Could you check a few things on this model? Use its own coordinates, in mm. Face numbers are marked on the shaded views. Give positions to 0.01 mm unless a question says otherwise; leave off trailing zeros. Write each loop counter-clockwise with the first axis right and the second up, starting at its lowest first coordinate (ties: lowest second). Pieces come first, ordered by that corner, then holes. Notation, with made-up numbers: (15, 65.5) - (49, 65.5) arc R18 ccw to (49, 97.5) - close; hole circle Ø9 at (19, 48). An arc over 180 degrees is marked (long way). Use one line per item in the form item = value.
Autodesk Inventor part; units mm, degrees
ref_plane "Work Plane2" through (0, 202, 0) normal (0, 1, 0) x (1, 0, 0)
ref_plane "YZ Plane" through (0, 0, 0) normal (1, 0, 0) x (0, 1, 0)
ref_plane "XZ Plane" through (0, 0, 0) normal (0, 1, 0) x (-1, 0, 0)
sketch "Sketch1" plane through (0, 0, 0) normal (0, 1, 0) x (-1, 0, 0)
  circle A0 centre (0, 0) radius 19.5
  circle A1 centre (0, 0) radius 18
  dimension "d0" = 39
  dimension "d1" = 36
extrude "Extrusion1" add sketch "Sketch1" along normal blind 182
ref_plane "Work Plane1" through (0, 192, 0) normal (0, 1, 0) x (1, 0, 0)
sketch "Sketch2" plane through (0, 192, 0) normal (0, 1, 0) x (1, 0, 0)
  circle A0 centre (0, 0) radius 5
  dimension "d5" = 10
loft "Loft1" add profiles "Sketch2" section 1 edges at (19.5, 182, 0)
sketch "Sketch3" plane through (0, 192, 0) normal (0, 1, 0) x (1, 0, 0)
  circle A0 centre (0, 0) radius 4
  dimension "d11" = 8
loft "Loft2" cut profiles "Sketch3" section 1 edges at (18, 182, 0)
sketch "Sketch4" plane through (0, 192, 0) normal (0, 1, 0) x (1, 0, 0)
  circle A0 centre (0, 0) radius 5
  circle A1 centre (0, 0) radius 4
  circle A2 centre (0, 0) radius 5
  dimension "d16" = 10
  dimension "d17" = 8
extrude "Extrusion2" add sketch "Sketch4" along normal blind 9
sketch "Sketch5" plane through (0, 192, 0) normal (0, 1, 0) x (1, 0, 0)
  circle A0 centre (0, 0) radius 4
  circle A1 centre (0, 0) radius 4
ref_plane "Work Plane2" through (0, 202, 0) normal (0, 1, 0) x (1, 0, 0)
sketch "Sketch6" plane through (0, 202, 0) normal (0, 1, 0) x (1, 0, 0)
  circle A0 centre (0, 0) radius 1.5
  line L0 (1.5, 0) -> (-1.5, 0) construction
  dimension "d21" = 3
extrude "Extrusion3" add sketch "Sketch5" along normal blind 3
extrude "Extrusion4" add sketch "Sketch6" against normal up to surface (7 mm away)
sketch "Sketch8" plane through (0, 202, 0) normal (0, 1, 0) x (1, 0, 0)
  circle A0 centre (0, 0) radius 1.5
  circle A1 centre (0, 0) radius 1
  dimension "d26" = 2
extrude "Extrusion5" cut sketch "Sketch8" against normal through all contours A1
thread "Thread1"
properties part number "xilanh" material "PMMA Plastic"
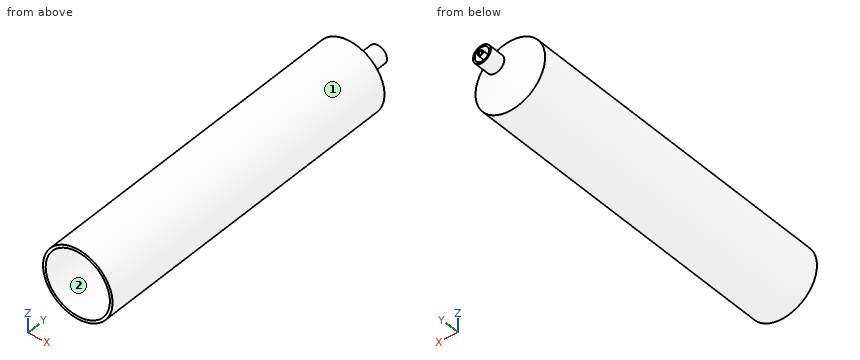
1. For pin 1 (9 mm diameter, centred on x = 1.5, z = 0.5, fed in from -Y); pin 2 (2 mm diameter, centred on y = 181.5, z = 9, fed in from -X); pin 3 (6.5 mm diameter, centred on x = -1.5, z = 0.5, fed in from +Y); pin 4 (10.5 mm diameter, centred on x = 0, z = 0, fed in from -Y), each with a flat end and sliding along its axis, tell me the tip position at first contact or that it passes through.
Response values:
pin_1 = 190.51
pin_2 = -17.78
pin_3 = 202
pin_4 = 191.11
2. If I drill on line 1 (Z direction, x = 0, y = 197); line 2 (Z direction, x = 0, y = 50.5), over which ranges is the centre line in solid material (lowest first)? Write a range as from..to.
Response values:
line_1 = -5..-4, -1.5..-1, 1..1.5, 4..5
line_2 = -19.5..-18, 18..19.5
3. Imagine slicing it at A-A, the plane y = 19. List the corners of the cut face in (x, z) for me.
Response values:
outline = circle Ø39 at (0, 0); hole circle Ø36 at (0, 0)
4. Imagine slicing it at B-B, the plane y = 187.5. List the corners of the cut face in (x, z) for me (3 decimals).
Response values:
outline = circle Ø23.05 at (0, 0); hole circle Ø20.6 at (0, 0)
5. If we mould it in two halves opening along Z, with no side actions, what happens to the marked faces 1 and 2? For each: pulls with the +Z half, pulls with the -Z half, needs draft (parallel to the pull), parting line crosses it, or undercut.
Response values:
face_1 = parting line crosses it
face_2 = undercut
